Design review of the part built by this model. Coordinates are the model's own, in mm. A direction names the side the tool comes from. Coordinates: 2 decimals unless noted, no trailing zeros. Loops run counter-clockwise (first coordinate to the right, second up) from the corner with the lowest first, then second, coordinate; pieces in that order, holes last.
Q1. Wall thickness on probe 1 along Y at (x, z) = (8.5, -8.5) (3 decimals); probe 2 along X at (y, z) = (-3, -5.5) (3 decimals); probe 3 along Z at (x, y) = (-4, -4.5): over which ranges is each line inside the solid? List them lowest first.
Q2. Add section C-C on y = -1.5. Give the boundary of the cut face in (x, z) (3 decimals), and give its area (3 significant figures).
Q3. Add section D-D on x = 6.5. Give the boundary of the cut face in (y, z) (3 decimals).
Q4. Add section B-B on x = -3. Give the boundary of the cut face in (y, z) (3 decimals), and give its area (3 significant figures).
Q5. For P1, Ø1.8, axis at x = 0.5, y = 0.5, coming from the -Z side; P2, Ø3, axis at x = -1.5, y = 2, coming from the -Z side, all flat-tipped, find the tip position at first contact; note any pin that passes through.
Q6. Add section A-A on z = -9. Give the boundary of the cut face in (x, y) (3 decimals), and give its area (3 significant figures).
Q7. Machinability: for faces 4 (the face through (0, -11.25, -5)), 5 (the face through (9.765, 0, -8)), which of the approach directions +Z, -Z, +X, -X, +Y, -Y give a long, thin tool a straight path to every point of the face, cutting with its end or side? Answer none if there is none.
Q8. Draft analysis for pull direction X (two halves, no side actions). For faces 1 (the face through (-0.1, -3, -4.5)), 2 (the face through (-15.06, 0, -5)), 3 (the face through (0, 0, 1.5)), state which applies: released by +X, released by -X, zero draft, split by the parting line, or undercut.
```python
from build123d import *

# Parameters (mm, degrees)
F0_W     = 30.12
F0_H     = 22.5
F1_DEPTH = 11.01
F2_W     = 19.53
F2_H     = 11.91
F3_DEPTH = 6.01
F4_W     = 11
F4_H     = 6
F5_DEPTH = 1
F6_DEPTH = 1.5


with BuildPart() as f1:
    # F0 (on Top) → F1 (new body)
    with BuildSketch(Plane.XY):
        Rectangle(F0_W, F0_H)
    extrude(amount=-F1_DEPTH)

    # F2 (on face) → F3 (cut)
    with BuildSketch(Plane(origin=(0, 0, -11.01), x_dir=(1, 0, 0), z_dir=(0, 0, -1))):
        Rectangle(F2_W, F2_H)
    extrude(amount=-F3_DEPTH, mode=Mode.SUBTRACT)

    # F4 (on face) → F5 (cut)
    with BuildSketch(Plane(origin=(0, 0, -5), x_dir=(1, 0, 0), z_dir=(0, 0, -1))):
        Rectangle(F4_W, F4_H)
    extrude(amount=-F5_DEPTH, mode=Mode.SUBTRACT)

    # F6 (add): a face of the model
    f6_faces = [f1.faces().sort_by_distance(p)[0] for p in [
        (0, 0, 0),
    ]]
    extrude(f6_faces, amount=F6_DEPTH)


solid = f1.part
```
Entries:
1. probe 1: y = -11.25 to -5.955, 5.955 to 11.25
1. probe 2: x = -15.06 to -9.765, 9.765 to 15.06
1. probe 3: z = -5 to 1.5
2. outline: (-15.06, -11.01) - (-9.765, -11.01) - (-9.765, -5) - (-5.5, -5) - (-5.5, -4) - (5.5, -4) - (5.5, -5) - (9.765, -5) - (9.765, -11.01) - (15.06, -11.01) - (15.06, 1.5) - (-15.06, 1.5) - close
2. area: 248 mm2
3. outline: (-11.25, -11.01) - (-5.955, -11.01) - (-5.955, -5) - (5.955, -5) - (5.955, -11.01) - (11.25, -11.01) - (11.25, 1.5) - (-11.25, 1.5) - close
4. outline: (-11.25, -11.01) - (-5.955, -11.01) - (-5.955, -5) - (-3, -5) - (-3, -4) - (3, -4) - (3, -5) - (5.955, -5) - (5.955, -11.01) - (11.25, -11.01) - (11.25, 1.5) - (-11.25, 1.5) - close
4. area: 204 mm2
5. P1: stops at z = -4
5. P2: stops at z = -5
6. outline: (-15.06, -11.25) - (15.06, -11.25) - (15.06, 11.25) - (-15.06, 11.25) - close; hole (-9.765, -5.955) - (9.765, -5.955) - (9.765, 5.955) - (-9.765, 5.955) - close
6. area: 445 mm2
7. face 4: +Z, -Z, +X, -X, -Y
7. face 5: -Z
8. face 1: undercut
8. face 2: released by -X
8. face 3: zero draft
